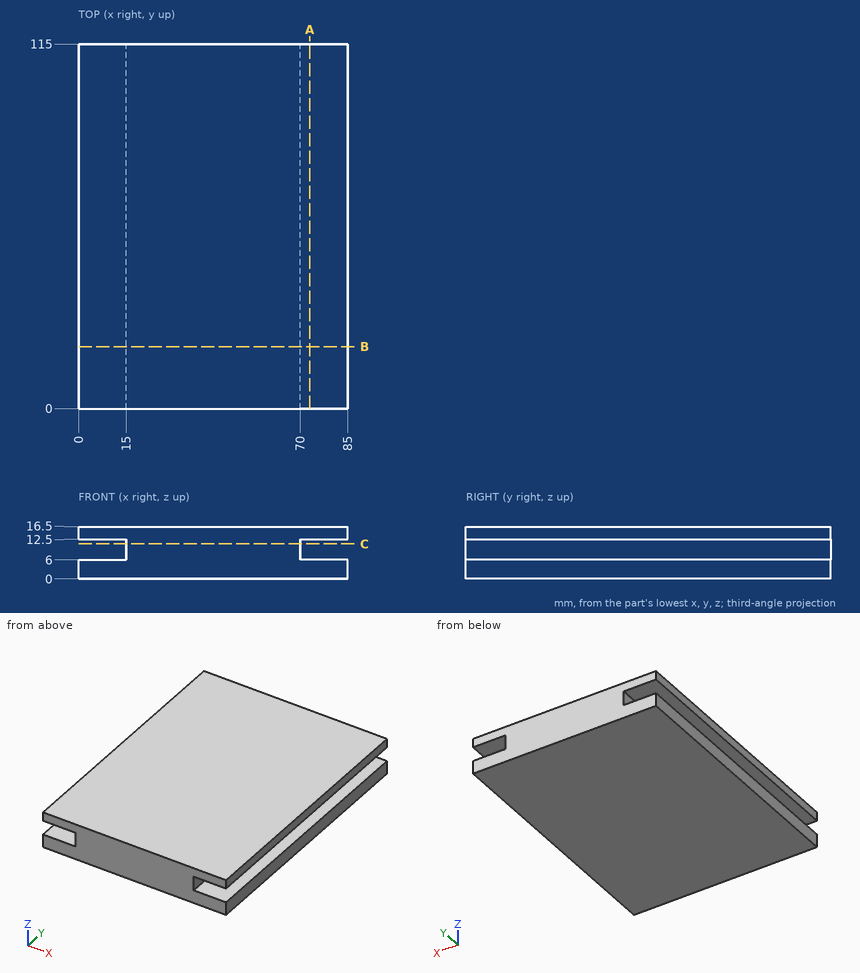
The drawing under review shows one solid part. Ordinate dimensions are in mm from its lowest x, y, z. Coordinates: 2 decimals unless noted, no trailing zeros. Write each loop counter-clockwise with the first axis right and the second up, starting at its lowest first coordinate (ties: lowest second). Pieces come first, ordered by that corner, then holes. Notation, with made-up numbers: (54.25, -38) -> (98.25, -38) arc R29 ccw to (98.25, -6) -> close; hole circle Ø3 at (82, 34). An arc over 180 degrees is marked (long way). Write each question's results on one line, items separated by ' | '. Start each with the question number.
1) Consider section B-B (y = 19.5). Write out the cut boundary in (x, z), plus the area to 3 significant figures.
2) Insertion check: pin 1 (3 mm diameter, centred on y = 31, z = 8.5, fed in from +X). The pin has a flat end and moves straight along its axis. Give the tip position at first contact, or say it passes through.
3) Consider section A-A (x = 73). Write out the cut boundary in (y, z).
4) Wall thickness on L1, parallel to Z at x = 71, y = 41.5; L2, parallel to X at y = 32.5, z = 7: over which ranges is each line inside the solid? List them lowest first. Write a range as [from, to].
5) Consider section C-C (z = 11). Write out the cut boundary in (x, y).
Geometry says:
1) outline: (0, 0) -> (85, 0) -> (85, 6) -> (70, 6) -> (70, 12.5) -> (85, 12.5) -> (85, 16.5) -> (0, 16.5) -> (0, 12.5) -> (15, 12.5) -> (15, 6) -> (0, 6) -> close | area: 1,210 mm^2
2) pin 1: x = 70
3) outline: (0, 0) -> (115, 0) -> (115, 6) -> (0, 6) -> close; (0, 12.5) -> (115, 12.5) -> (115, 16.5) -> (0, 16.5) -> close
4) L1: [0, 6], [12.5, 16.5] | L2: [15, 70]
5) outline: (15, 0) -> (70, 0) -> (70, 115) -> (15, 115) -> close
